from build123d import *

# Parameters (mm, degrees)
BOSS_EXTRUDE1_DEPTH = 3.175
SKETCH2_R           = 2.032
CUT_EXTRUDE1_DEPTH  = 242.929632893
FILLET1_R           = 12.7
FILLET2_R           = 0.79375
FILLET3_R           = 6.35
BOSS_EXTRUDE2_DEPTH = 6.35
CUT_EXTRUDE2_DEPTH  = 242.929633019


with BuildPart() as part:
    # Sketch1 → Boss-Extrude1 (new, symmetric)
    with BuildSketch(Plane(origin=(0, 0, 0), x_dir=(0, 0, -1), z_dir=(1, 0, 0))):
        with BuildLine():
            Line((-17.7, 19.05), (-17.7, 183.35625))
            ThreePointArc((-17.7, 183.35625), (-18.132742006, 186.643251873), (-19.401477372, 189.70625))
            Line((-19.401477372, 189.70625), (-34.524445986, 215.9))
            ThreePointArc((-34.524445986, 215.9), (-45.522968614, 222.25), (-56.521491242, 215.9))
            ThreePointArc((-56.521491242, 215.9), (-63.027187227, 214.156804014), (-64.770383213, 220.6625))
            ThreePointArc((-64.770383213, 220.6625), (-43.689881509, 232.833333333), (-22.609379805, 220.6625))
            Line((-22.609379805, 220.6625), (-1.825, 184.662898174))
            Line((-1.825, 184.662898174), (17.656128594, 19.795145732))
            ThreePointArc((17.656128594, 19.795145732), (16.917823934, 15.996831704), (14.112111824, 13.332199875))
            ThreePointArc((14.112111824, 13.332199875), (9.73081975, 6.35), (14.112111824, -0.632199875))
            ThreePointArc((14.112111824, -0.632199875), (17.067800125, -9.112111824), (8.587888176, -12.067800125))
            ThreePointArc((8.587888176, -12.067800125), (-0.205881062, -12.332007866), (-5.032111824, -19.687800125))
            ThreePointArc((-5.032111824, -19.687800125), (-11.987800125, -25.367888176), (-17.667888176, -18.412199875))
            ThreePointArc((-17.667888176, -18.412199875), (-16.740874674, 0), (-17.667888176, 18.412199875))
            ThreePointArc((-17.667888176, 18.412199875), (-17.691966963, 18.730696003), (-17.7, 19.05))
        make_face()
        with BuildLine():
            Line((-11.35, 25.4), (-11.35, 69.85))
            Line((-11.35, 69.85), (10.604854268, 25.356128594))
            ThreePointArc((10.604854268, 25.356128594), (9.571869946, 25.145962066), (8.587888176, 24.767800125))
            ThreePointArc((8.587888176, 24.767800125), (0, 22.802180275), (-8.587888176, 24.767800125))
            ThreePointArc((-8.587888176, 24.767800125), (-9.933230928, 25.239932584), (-11.35, 25.4))
        make_face(mode=Mode.SUBTRACT)
        Polygon((9.490062912, 34.790548391), (-11.35, 77.025175321), (4.499528462, 77.025175321), align=None, mode=Mode.SUBTRACT)
        Polygon((4.124363626, 80.200175321), (-11.35, 80.200175321), (-11.35, 111.560636058), align=None, mode=Mode.SUBTRACT)
        Polygon((3.00957227, 89.634595118), (-11.35, 118.735811379), (-0.429090099, 118.735811379), align=None, mode=Mode.SUBTRACT)
        Polygon((-0.804254935, 121.910811379), (-11.35, 121.910811379), (-11.35, 143.282896982), align=None, mode=Mode.SUBTRACT)
        with BuildLine():
            Line((-8.185967852, 184.381854159), (-1.919046291, 131.345231176))
            Line((-1.919046291, 131.345231176), (-11.35, 150.458072303))
            Line((-11.35, 150.458072303), (-11.35, 184.195567726))
            ThreePointArc((-11.35, 184.195567726), (-9.855804513, 185.780323391), (-8.185967852, 184.381854159))
        make_face(mode=Mode.SUBTRACT)
    extrude(amount=BOSS_EXTRUDE1_DEPTH, both=True)

    # Sketch2 → Cut-Extrude1 (cut, through all)
    with BuildSketch(Plane(origin=(3.175, 0, 0), x_dir=(0, 0, -1), z_dir=(1, 0, 0))):
        with Locations((11.35, -6.35)):
            Circle(SKETCH2_R)
        with Locations((11.35, 19.05)):
            Circle(SKETCH2_R)
        with Locations((-11.35, 19.05)):
            Circle(SKETCH2_R)
        with Locations((-11.35, -19.05)):
            Circle(SKETCH2_R)
    extrude(amount=-CUT_EXTRUDE1_DEPTH, mode=Mode.SUBTRACT)

    # Fillet1
    fillet1_edges = [part.edges().sort_by_distance(p)[0] for p in [
        (0, 184.662898174, 1.825),
    ]]
    fillet(fillet1_edges, radius=FILLET1_R)

    # Fillet2
    fillet2_edges = [part.edges().sort_by_distance(p)[0] for p in [
        (0, 69.85, 11.35),
        (0, 34.790548391, -9.490062912),
        (0, 77.025175321, -4.499528462),
        (0, 77.025175321, 11.35),
        (0, 80.200175321, -4.124363626),
        (0, 111.560636058, 11.35),
        (0, 80.200175321, 11.35),
        (0, 89.634595118, -3.00957227),
        (0, 118.735811379, 0.429090099),
        (0, 118.735811379, 11.35),
        (0, 121.910811379, 0.804254935),
        (0, 143.282896982, 11.35),
        (0, 121.910811379, 11.35),
        (0, 150.458072303, 11.35),
        (0, 131.345231176, 1.919046291),
    ]]
    fillet(fillet2_edges, radius=FILLET2_R)

    # Fillet3
    fillet3_edges = [part.edges().sort_by_distance(p)[0] for p in [
        (0, 25.4, 11.35),
        (0, 25.356128594, -10.604854268),
    ]]
    fillet(fillet3_edges, radius=FILLET3_R)

    # Sketch3 → Boss-Extrude2 (add)
    with BuildSketch(Plane(origin=(3.175, 0, 0), x_dir=(0, 0, -1), z_dir=(1, 0, 0))):
        with BuildLine():
            Line((-17.7, 113.663160513), (-17.7, 90.742041294))
            Line((-17.7, 90.742041294), (-40.826076924, 106.814372593))
            ThreePointArc((-40.826076924, 106.814372593), (-47.50636364, 107.166070544), (-50.794697112, 101.340541809))
            ThreePointArc((-50.794697112, 101.340541809), (-52.976424691, 98.851804162), (-55.570143469, 100.907618649))
            ThreePointArc((-55.570143469, 100.907618649), (-45.805288512, 120.644406163), (-23.869094131, 118.721764812))
            Line((-23.869094131, 118.721764812), (-17.7, 113.663160513))
        make_face()
    extrude(amount=-BOSS_EXTRUDE2_DEPTH)

    # Sketch4 → Cut-Extrude2 (cut, through all)
    with BuildSketch(Plane(origin=(3.175, 0, 0), x_dir=(0, 0, -1), z_dir=(1, 0, 0))):
        Polygon((-17.7, 98.474994642), (-32.722386581, 108.91536353), (-32.722386581, 120.21942978), (-17.7, 120.21942978), align=None)
    extrude(amount=-CUT_EXTRUDE2_DEPTH, mode=Mode.SUBTRACT)


solid = part.part
CAD build for the part. Positions are in the model's coordinates, mm. A direction names the side the tool comes from. Give positions to 0.01 mm unless a question says otherwise; leave off trailing zeros. Loops run counter-clockwise (first coordinate to the right, second up) from the corner with the lowest first, then second, coordinate; pieces in that order, holes last. Notation, with made-up numbers: M 16,54.25 L 47,54.25 A26 ccw 47,79.25 Z; hole C -23,47 d6. An arc over 180 degrees is marked long. Answer in a Markdown table with one row per item. Add a question column.
Item 1: Band-saw the part on D-D on x = -2. Give the number of separate pieces and of enclosed holes in the cut face, then the cut area to 3 significant figures.
Item 2: Band-saw the part on C-C on z = 43. Give the cut face in (x, y) (3 decimals), then the cut area to 3 significant figures.
Item 3: Tool access for faces 1 (the face through (0.044, 160.494, 5.363)), 2 (the face through (0.04, 6.47, -9.73)), 3 (the face through (0, 54, 17.7)), 4 (the face through (0.04, 186.6, 18.12)): list every direction of +Z, -Z, +X, -X, +Y, -Y with a clear straight run to the whole face (end or side of a thin tool).
Item 4: Probe probe 1 along Z at (x, y) = (1.25, 113.5); probe 2 along Y at (x, z) = (-2.5, 39); probe 3 along Z at (x, y) = (0.5, 55.5). List the from-to ranges inside material, lowest first.
Item 5: Drop flat-ended pins along their axis: P1, Ø1.9, axis at x = -0.5, y = 154.5, coming from the +Z side; P2, Ø3, axis at x = -1.5, y = 127, coming from the -Z side; P3, Ø12, axis at y = 9, z = 24.5, coming from the -X side; P4, Ø1, axis at x = 0, z = 33.5, coming from the +Y side. Give the stop position or say it passes through.
Item 6: Mould opens along Y. For faces 5 (the face through (0, 167, 11.35)), 6 (the face through (3.175, 104, 14)), 7 (the face through (0.04, -12.27, 0.09)) say: +Y half, -Y half, draft (parallel to the pull), parting line (faces both ways), or undercut.
Item 7: Band-saw the part on A-A on y = 129. Give the cut face in (x, z) (3 decimals), then the cut area to 3 significant figures.
Item 8: Band-saw the part on B-B on z = 28.5. Give the cut face in (x, y) (3 decimals).
Reply:
| question | item | result |
|---|---|---|
| 1 | separate pieces | 1 |
| 1 | enclosed holes | 10 |
| 1 | area | 5,170 mm^2 |
| 2 | outline | M -3.175,107.782 L 3.175,107.782 L 3.175,121.94 L -3.175,121.94 Z; M -3.175,221.997 L 3.175,221.997 L 3.175,232.824 L -3.175,232.824 Z |
| 2 | area | 159 mm^2 |
| 3 | face 1 | +X, -X |
| 3 | face 2 | -Z, +X, -X |
| 3 | face 3 | +Z, +X, -X, -Y |
| 3 | face 4 | +Z, +X, -X |
| 4 | probe 1 | z = -6.58 to -0.19, 8.77 to 17.7, 32.72 to 53.08 |
| 4 | probe 2 | y = 105.55 to 122.95, 220.45 to 232.38 |
| 4 | probe 3 | z = -13.44 to -7.04, 0.73 to 4.27, 11.35 to 17.7 |
| 5 | P1 | stops at z = 17.7 |
| 5 | P2 | stops at z = -5.17 |
| 5 | P3 | passes through |
| 5 | P4 | stops at y = 230.82 |
| 6 | face 5 | undercut |
| 6 | face 6 | draft |
| 6 | face 7 | -Y half |
| 7 | outline | M -3.175,-4.752 L 3.175,-4.752 L 3.175,4.302 L -3.175,4.302 Z; M -3.175,11.35 L 3.175,11.35 L 3.175,17.7 L -3.175,17.7 Z |
| 7 | area | 97.8 mm^2 |
| 8 | outline | M -3.175,98.248 L 3.175,98.248 L 3.175,105.981 L -3.175,105.981 Z; M -3.175,120.219 L 3.175,120.219 L 3.175,121.545 L -3.175,121.545 Z; M -3.175,205.465 L 3.175,205.465 L 3.175,227.512 L -3.175,227.512 Z |
